Could you check a few things on this model? Use its own coordinates, in mm. A direction names the side the tool comes from. Round coordinates to 2 decimals unless told otherwise and drop trailing zeros. Loops run counter-clockwise (first coordinate to the right, second up) from the corner with the lowest first, then second, coordinate; pieces in that order, holes last. Notation, with made-up numbers: (-25, 35) -> (-13, 35) arc R23 ccw to (-13, 57) -> close; hole circle Ø5 at (-6, 53). An arc over 180 degrees is marked (long way). One line per item, written item: value.
```python
from build123d import *

# Parameters (mm, degrees)
SKETCH1_W           = 80.6
SKETCH1_H           = 36
BOSS_EXTRUDE1_DEPTH = 1
SKETCH2_W           = 69
SKETCH2_H           = 24
BOSS_EXTRUDE2_DEPTH = 7.4
SKETCH3_R           = 1.5
CUT_EXTRUDE1_DEPTH  = 7.4
SKETCH4_W           = 67
SKETCH4_H           = 22
CUT_EXTRUDE2_DEPTH  = 2
CUT_EXTRUDE2_DRAFT  = -15


with BuildPart() as part:
    # Sketch1 → Boss-Extrude1 (new body)
    with BuildSketch(Plane(origin=(0, 0, 0), x_dir=(1, 0, 0), z_dir=(0, 1, 0))):
        with Locations((40.3, 18)):
            Rectangle(SKETCH1_W, SKETCH1_H)
    extrude(amount=BOSS_EXTRUDE1_DEPTH)

    # Sketch2 → Boss-Extrude2 (add)
    with BuildSketch(Plane(origin=(0, 1, 0), x_dir=(1, 0, 0), z_dir=(0, 1, 0))):
        with Locations((40.3, 18)):
            Rectangle(SKETCH2_W, SKETCH2_H)
    extrude(amount=BOSS_EXTRUDE2_DEPTH)

    # Sketch3 → Cut-Extrude1 (cut)
    with BuildSketch(Plane(origin=(0, 1, 0), x_dir=(1, 0, 0), z_dir=(0, 1, 0))):
        with Locations(Location((3.1, 33.5, 0), (0, 0, 270))):
            Circle(SKETCH3_R)
        with Locations(Location((3.1, 2.5, 0), (0, 0, 270))):
            Circle(SKETCH3_R)
        with Locations(Location((78.1, 2.5, 0), (0, 0, 270))):
            Circle(SKETCH3_R)
        with Locations(Location((78.1, 33.5, 0), (0, 0, 270))):
            Circle(SKETCH3_R)
    extrude(amount=-CUT_EXTRUDE1_DEPTH, mode=Mode.SUBTRACT)


with BuildPart() as cut_extrude2_tool:
    # Sketch4 → Cut-Extrude2 (with draft: the straight prism first)
    with BuildSketch(Plane(origin=(0, 8.4, 0), x_dir=(1, 0, 0), z_dir=(0, 1, 0))):
        with Locations((40.3, 18)):
            Rectangle(SKETCH4_W, SKETCH4_H)
    extrude(amount=-CUT_EXTRUDE2_DEPTH)
    # Cut-Extrude2: the draft: its side faces are tilted about the plane it starts from
    cut_extrude2_sides = [cut_extrude2_tool.faces().sort_by_distance(p)[0] for p in [
        (6.8, 7.4, -18),
        (40.3, 7.4, -7),
        (73.8, 7.4, -18),
        (40.3, 7.4, -29),
    ]]
    draft(cut_extrude2_sides, Plane(origin=(0, 8.4, 0), x_dir=(1, 0, 0), z_dir=(0, 1, 0)), CUT_EXTRUDE2_DRAFT)


with BuildPart() as part_1:
    add(part.part)

    # Cut-Extrude2: cut by cut_extrude2_tool
    add(cut_extrude2_tool.part, mode=Mode.SUBTRACT)


solid = part_1.part
```
Item 1: If we section it at B-B on z = -2.5: List the corners of the cut face in (x, y) for me, plus the area to 3 significant figures.
Output:
outline: (0, 0) -> (1.6, 0) -> (1.6, 1) -> (0, 1) -> close; (4.6, 0) -> (76.6, 0) -> (76.6, 1) -> (4.6, 1) -> close; (79.6, 0) -> (80.6, 0) -> (80.6, 1) -> (79.6, 1) -> close
area: 74.6 mm²
Item 2: For faces 1 (the face through (7.064, 7.414, -17.846)), 2 (the face through (40, 5, -6)), 3 (the face through (74.8, 5, -18)), which set-ups out of +Z, -Z, +X, -X, +Y, -Y let a thin tool reach every point of the face, with its end or its side?
Output:
face 1: +Y
face 2: +Z, +X, -X, +Y
face 3: +Z, -Z, +X, +Y
Item 3: Will these pins go through, and if not, where does the flat tip stop? pin 1 Ø4 at (x, y) = (64.5, 6) entering from -Z; pin 2 Ø6.5 at (x, z) = (56.5, -16.5) entering from +Y; pin 3 Ø5 at (x, z) = (78.1, -33.5) entering from +Y.
Output:
pin 1: stops at z = -30
pin 2: stops at y = 6.4
pin 3: stops at y = 1
Item 4: If we mould it in two halves opening along Z, with no side actions, what happens to faces 4 (the face through (39.831, 7.414, -28.736)), 5 (the face through (40, 5, -30)), 6 (the face through (5.8, 5, -18))? For each: released by +Z, released by -Z, zero draft, split by the parting line, or undercut.
Output:
face 4: undercut
face 5: released by -Z
face 6: zero draft
Item 5: If we section it at A-A on x = 78.1: List the corners of the cut face in (y, z) for me, plus the area to 3 significant figures.
Output:
outline: (0, -36) -> (1, -36) -> (1, -35) -> (0, -35) -> close; (0, -32) -> (1, -32) -> (1, -4) -> (0, -4) -> close; (0, -1) -> (1, -1) -> (1, 0) -> (0, 0) -> close
area: 30.0 mm²
Item 6: I need wall thicknesses on line 1 (X direction, y = 0.6, z = -2.5); line 2 (Z direction, x = 78.1, y = 0.7); line 3 (Y direction, x = 50, z = -8). Which ranges of each line are inside material? Lowest first, please. Write a range as from..to.
Output:
line 1: x = 0..1.6, 4.6..76.6, 79.6..80.6
line 2: z = -36..-35, -32..-4, -1..0
line 3: y = 0..6.4
Item 7: If we section it at C-C on x = 66: List the corners of the cut face in (y, z) for me, plus the area to 3 significant figures.
Output:
outline: (0, -36) -> (1, -36) -> (1, -30) -> (8.4, -30) -> (8.4, -29) -> (6.4, -28.46) -> (6.4, -7.54) -> (8.4, -7) -> (8.4, -6) -> (1, -6) -> (1, 0) -> (0, 0) -> close
area: 171 mm²
Item 8: If we section it at D-D on y = 3.5: List the corners of the cut face in (x, z) for me.
Output:
outline: (5.8, -30) -> (74.8, -30) -> (74.8, -6) -> (5.8, -6) -> close
